Geometry: final body of the model. Coordinates: model frame, mm. Face numbers are marked on the shaded views. A direction names the side the tool comes from. Give positions to 0.01 mm unless a question says otherwise; leave off trailing zeros. Order: outer loops, then holes, each group sorted by start corner. A loop starts at its lowest first (then second) coordinate and runs counter-clockwise, first axis right, second up. Notation, with made-up numbers: (-16, 15.25) -> (-5, 15.25) arc R13 ccw to (-5, 26.25) -> close; hole circle Ø5 at (41.25, 37). An arc over 180 degrees is marked (long way). One line per question, with ' | ' between items. Start each with the question number.
(1) Section B-B (x = -19.5). Return loops of the section in (y, z), then the cut area to 3 significant figures.
(2) Section A-A (y = 10.5). Return loops of the section in (x, z).
(3) First-contact query: pin 1 Ø6 at (x, y) = (-10.5, -2) entering from -Z; pin 2 Ø7 at (x, y) = (-9, 16.5) entering from +Z; pin 3 Ø12 at (y, z) = (0, 17.5) entering from +X; pin 4 Ø7.5 at (y, z) = (2, 10) entering from -X. Flat tips, straight axial feed; report the tip coordinate or a pass-through.
(4) Mould query, pull axis Z, two halves, no side actions, for the marked faces 1, 2 and 3. Classes: +Z half, -Z half, draft (parallel to the pull), parting line (faces both ways), or undercut.
(5) Ray query, L1, parallel to Y at x = 12, z = 14.5; L2, parallel to X at y = -10.75, z = 57.3; L3, parallel to Y at x = -12.5, z = 55. Return the intervals inside material, ascending.
(6) Section C-C (z = 51). Return loops of the section in (x, y), then the cut area to 3 significant figures.
(7) Set-up query: the marked faces 4, 5, 6 and 7. Return all of +Z, -Z, +X, -X, +Y, -Y with unobstructed straight access to the full face (end or side cutting, diameter ignored); none if empty.
(8) Section D-D (y = 1.25). Return loops of the section in (x, z), then the cut area to 3 significant figures.
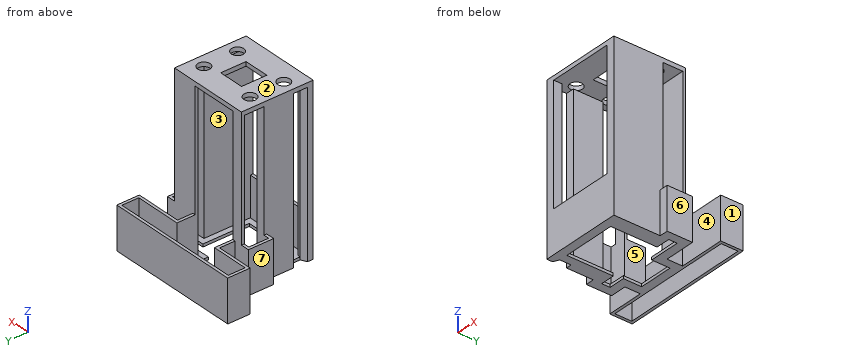
```python
from build123d import *

# Parameters (mm, degrees)
EXTRUDE_1_DEPTH        = 15
CUT_EXTRUDE_1_DEPTH    = 14
SKETCH_7_W             = 46
SKETCH_7_H             = 6
CUT_EXTRUDE_2_DEPTH    = 1
SKETCH_8_W             = 14
SKETCH_8_H             = 4
CUT_EXTRUDE_3_DEPTH    = 1
CUT_EXTRUDE_6_DEPTH    = 1
EXTRUDE_START          = -57
EXTRUDE_10_OUTLINE_W   = 3
EXTRUDE_10_OUTLINE_H   = 17.5
EXTRUDE_10_OUTLINE_H_2 = 10.5
EXTRUDE_10_OUTLINE_W_2 = 9
EXTRUDE_10_OUTLINE_H_3 = 1
EXTRUDE_10_OUTLINE_W_3 = 2
EXTRUDE_10_DEPTH       = 57
SKETCH_29_W            = 29
SKETCH_29_H            = 25.5
EXTRUDE_12_DEPTH       = 1.5
SKETCH_30_R            = 2.2
SKETCH_30_W            = 9
SKETCH_30_H            = 9
CUT_EXTRUDE_8_DEPTH    = 1.5
SKETCH_31_W            = 1.75
SKETCH_31_H            = 1
EXTRUDE_13_DEPTH       = 42


# Read off the part's stored shape, not the designer's step: 凸台-拉伸10
with BuildPart() as part:
    # 草图3 → 凸台-拉伸1 (new body)
    with BuildSketch(Plane.XY):
        Polygon((-25, 21.5), (23, 21.5), (23, 13.5), (6.5, 13.5), (6.5, 8), (17.5, 8), (17.5, -1), (12.5, -1), (12.5, -17.5), (-12.5, -17.5), (-12.5, -1), (-17.5, -1), (-17.5, 8), (-11.75, 8), (-11.75, 13.5), (-25, 13.5), align=None)
    extrude(amount=EXTRUDE_1_DEPTH)

    # 草图4 → 切除-拉伸1 (cut)
    with BuildSketch(Plane.XY.offset(15)):
        Polygon((22, 20.5), (-24, 20.5), (-24, 14.5), (-10.75, 14.5), (-10.75, 7), (-16.5, 7), (-16.5, 0), (-11.5, 0), (-11.5, -16.5), (11.5, -16.5), (11.5, 0), (16.5, 0), (16.5, 7), (5.5, 7), (5.5, 14.5), (22, 14.5), align=None)
    extrude(amount=-CUT_EXTRUDE_1_DEPTH, mode=Mode.SUBTRACT)

    # 草图7 → 切除-拉伸2 (cut)
    with BuildSketch(Plane.XY.offset(1)):
        with Locations((-1, 17.5)):
            Rectangle(SKETCH_7_W, SKETCH_7_H)
    extrude(amount=-CUT_EXTRUDE_2_DEPTH, mode=Mode.SUBTRACT)

    # 草图8 → 切除-拉伸3 (cut)
    with BuildSketch(Plane.ZY.offset(12.5)):
        with Locations((8, -12.5)):
            Rectangle(SKETCH_8_W, SKETCH_8_H)
    extrude(amount=-CUT_EXTRUDE_3_DEPTH, mode=Mode.SUBTRACT)

    # 草图9 → 切除-拉伸6 (cut)
    with BuildSketch(Plane(origin=(0, 0, 0), x_dir=(-1, 0, 0), z_dir=(0, 0, -1))):
        Polygon((-3.5, 11.5), (-3.5, 5), (-14.5, 5), (-14.5, 2), (-9.5, 2), (-9.5, -14.5), (9.5, -14.5), (9.5, 2), (14.5, 2), (14.5, 5), (8.75, 5), (8.75, 11.5), align=None)
    extrude(amount=-CUT_EXTRUDE_6_DEPTH, mode=Mode.SUBTRACT)

    # 凸台-拉伸10 outline → 凸台-拉伸10 (add)
    with BuildSketch(Plane(origin=(0, 0, 0), x_dir=(-1, 0, 0), z_dir=(0, 0, -1)).offset(EXTRUDE_START)):
        with Locations((-13, -8.75)):
            Rectangle(EXTRUDE_10_OUTLINE_W, EXTRUDE_10_OUTLINE_H)
        Polygon((14.5, -15.5), (12.5, -14.5), (11.5, -14.5), (11.5, -17.5), (14.5, -17.5), align=None)
        with Locations((13, -5.25)):
            Rectangle(EXTRUDE_10_OUTLINE_W, EXTRUDE_10_OUTLINE_H_2)
        with Locations((-10, 7.5)):
            Rectangle(EXTRUDE_10_OUTLINE_W_2, EXTRUDE_10_OUTLINE_H_3)
        with Locations((13.5, 7.5)):
            Rectangle(EXTRUDE_10_OUTLINE_W_3, EXTRUDE_10_OUTLINE_H_3)
    extrude(amount=EXTRUDE_10_DEPTH)

    # 草图29 → 凸台-拉伸12 (add)
    with BuildSketch(Plane.XY.offset(57)):
        with Locations((0, -4.75)):
            Rectangle(SKETCH_29_W, SKETCH_29_H)
    extrude(amount=EXTRUDE_12_DEPTH)

    # 草图30 → 切除-拉伸8 (cut)
    with BuildSketch(Plane.XY.offset(58.5)):
        with Locations((-10, 1.25)):
            Circle(SKETCH_30_R)
        with Locations((-10, -10.75)):
            Circle(SKETCH_30_R)
        with Locations((10, 1.25)):
            Circle(SKETCH_30_R)
        with Locations((10, -10.75)):
            Circle(SKETCH_30_R)
        with Locations((0, -4.75)):
            Rectangle(SKETCH_30_W, SKETCH_30_H)
    extrude(amount=-CUT_EXTRUDE_8_DEPTH, mode=Mode.SUBTRACT)

    # 草图31 → 凸台-拉伸13 (add)
    with BuildSketch(Plane.XY.offset(15)):
        with Locations((-11.625, 7.5)):
            Rectangle(SKETCH_31_W, SKETCH_31_H)
    extrude(amount=EXTRUDE_13_DEPTH)


solid = part.part
```
Response:
1) outline: (13.5, 0) -> (14.5, 0) -> (14.5, 15) -> (13.5, 15) -> close; (20.5, 0) -> (21.5, 0) -> (21.5, 15) -> (20.5, 15) -> close | area: 30.0 mm^2
2) outline: (-11.75, 0) -> (-8.75, 0) -> (-8.75, 1) -> (-10.75, 1) -> (-10.75, 15) -> (-11.75, 15) -> close; (3.5, 0) -> (6.5, 0) -> (6.5, 15) -> (5.5, 15) -> (5.5, 1) -> (3.5, 1) -> close
3) pin 1: stops at z = 0 | pin 2: stops at z = 15 | pin 3: stops at x = 17.5 | pin 4: stops at x = -17.5
4) face 1: draft | face 2: +Z half | face 3: undercut
5) L1: y = -17.5 to 0, 7 to 8, 13.5 to 14.5, 20.5 to 21.5 | L2: x = -14.5 to -12.2, -7.8 to 7.8, 12.2 to 14.5 | L3: y = -17.5 to -14.5, -10.5 to 0, 7 to 8
6) outline: (-14.5, -17.5) -> (-11.5, -17.5) -> (-11.5, -14.5) -> (-12.5, -14.5) -> (-14.5, -15.5) -> close; (-14.5, -10.5) -> (-11.5, -10.5) -> (-11.5, 0) -> (-14.5, 0) -> close; (-14.5, 7) -> (-10.75, 7) -> (-10.75, 8) -> (-14.5, 8) -> close; (5.5, 7) -> (14.5, 7) -> (14.5, 8) -> (5.5, 8) -> close; (11.5, -17.5) -> (14.5, -17.5) -> (14.5, 0) -> (11.5, 0) -> close | area: 105 mm^2
7) face 4: +Z, -Z, +X | face 5: none | face 6: +Z, -Z, +X, -Y | face 7: +Z, -Z, -X, -Y
8) outline: (-17.5, 0) -> (-9.5, 0) -> (-9.5, 1) -> (-16.5, 1) -> (-16.5, 15) -> (-17.5, 15) -> close; (-14.5, 57) -> (-12.2, 57) -> (-12.2, 58.5) -> (-14.5, 58.5) -> close; (-7.8, 57) -> (7.8, 57) -> (7.8, 58.5) -> (-7.8, 58.5) -> close; (9.5, 0) -> (17.5, 0) -> (17.5, 15) -> (16.5, 15) -> (16.5, 1) -> (9.5, 1) -> close; (12.2, 57) -> (14.5, 57) -> (14.5, 58.5) -> (12.2, 58.5) -> close | area: 74.3 mm^2
